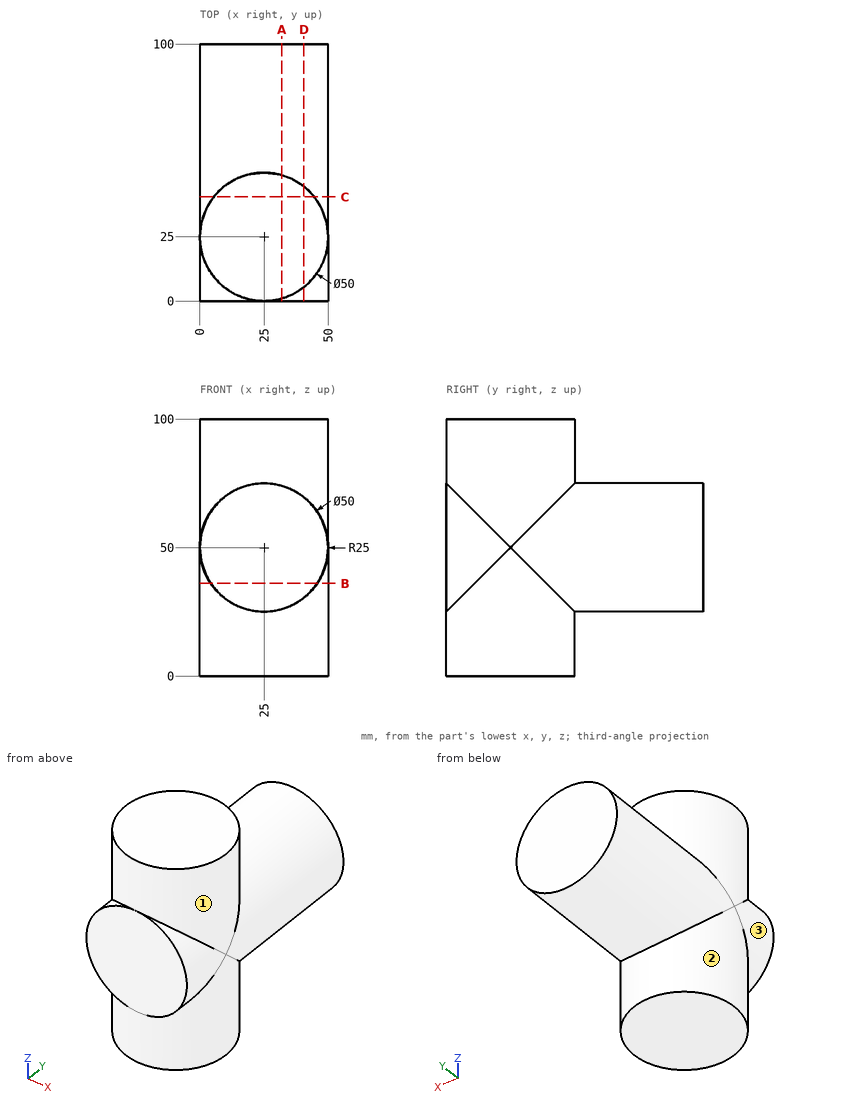
Geometry: see drawing. Coordinates: mm, zero at the bounding-box minimum. A direction names the side the tool comes from. Coordinates: 2 decimals unless noted, no trailing zeros. Loops run counter-clockwise (first coordinate to the right, second up) from the corner with the lowest first, then second, coordinate; pieces in that order, holes last. Notation, with made-up numbers: M 62,-9.5 L 114,-9.5 A23 cw 114,20.5 Z; hole C 45.25,-18 d1. An arc over 180 degrees is marked long. Answer in a Markdown table with one row per item.
Q1. Section A-A on x = 32. Return the cut outline in (y, z), plus the area to 3 significant figures.
Answers below:
| item | result |
|---|---|
| outline | M 0,26 L 1,26 L 1,0 L 49,0 L 49,26 L 100,26 L 100,74 L 49,74 L 49,100 L 1,100 L 1,74 L 0,74 Z |
| area | 7,300 mm^2 |
Q2. Set-up query: the marked faces 1, 2 and 3. Return all of +Z, -Z, +X, -X, +Y, -Y with unobstructed straight access to the full face (end or side cutting, diameter ignored); none if empty.
Answers below:
| item | result |
|---|---|
| face 1 | +Z |
| face 2 | -Z |
| face 3 | -X, -Y |
Q3. First-contact query: pin 1 (1.5 mm diameter, centred on x = 15, y = 49.5, fed in from -Z); pin 2 (2 mm diameter, centred on y = 50, z = 64, fed in from +X); pin 3 (3 mm diameter, centred on x = 12, y = 73.5, fed in from +Z); pin 4 (8 mm diameter, centred on y = 64, z = 81.5, fed in from -X). Flat tips, straight axial feed; report the tip coordinate or a pass-through.
Answers below:
| item | result |
|---|---|
| pin 1 | stops at z = 26.77 |
| pin 2 | stops at x = 46.35 |
| pin 3 | stops at z = 72.2 |
| pin 4 | passes through |
Q4. Section B-B on z = 36. Return the cut outline in (x, y), plus the area to 3 significant figures.
Answers below:
| item | result |
|---|---|
| outline | M 4.29,0 L 45.71,0 L 45.71,11 A25 ccw 45.71,39 L 45.71,100 L 4.29,100 L 4.29,39 A25 ccw 4.29,11 Z |
| area | 4,310 mm^2 |
Q5. Ray query, probe 1 along Z at (x, y) = (25, 79); probe 2 along X at (y, z) = (26, 78); probe 3 along X at (y, z) = (88, 34). Return the intervals inside material, ascending. Write a range as from..to.
Answers below:
| item | result |
|---|---|
| probe 1 | z = 25..75 |
| probe 2 | x = 0.02..49.98 |
| probe 3 | x = 5.79..44.21 |
Q6. Section D-D on x = 40.5. Return the cut outline in (y, z).
Answers below:
| item | result |
|---|---|
| outline | M 0,30.38 L 5.38,30.38 L 5.38,0 L 44.62,0 L 44.62,30.38 L 100,30.38 L 100,69.62 L 44.62,69.62 L 44.62,100 L 5.38,100 L 5.38,69.62 L 0,69.62 Z |
Q7. Section C-C on y = 40.5. Return the cut outline in (x, z), plus the area to 3 significant figures.
Answers below:
| item | result |
|---|---|
| outline | M 5.38,0 L 44.62,0 L 44.62,34.5 A25 ccw 44.62,65.5 L 44.62,100 L 5.38,100 L 5.38,65.5 A25 ccw 5.38,34.5 Z |
| area | 4,150 mm^2 |
